from build123d import *

# Parameters (mm, degrees)
EXTRU_MINCE1_DEPTH      = 38
BOSS_EXTRU_1_DEPTH      = 1.2
CONG_1_R                = 1
BOSS_EXTRU_2_DEPTH      = 12
ESQUISSE4_R             = 1.5
ENL_V_MAT_EXTRU_1_DEPTH = 68.523625665
ESQUISSE5_W             = 8.01820663
ESQUISSE5_H             = 8
ENL_V_MAT_EXTRU_2_DEPTH = 10
CONG_2_R                = 3


with BuildPart() as part:
    # Esquisse1 → Extru.-Mince1 (new body)
    with BuildSketch(Plane(origin=(0, 0, 0), x_dir=(1, 0, 0), z_dir=(0, 1, 0))):
        with BuildLine():
            ThreePointArc((19.5687881, -17.869318182), (0, 26.5), (-19.5687881, -17.869318182))
            ThreePointArc((-19.5687881, -17.869318182), (0, -2), (19.5687881, -17.869318182))
        make_face()
        with BuildLine():
            ThreePointArc((20.124375889, -15.332954545), (0, 25.3), (-20.124375889, -15.332954545))
            ThreePointArc((-20.124375889, -15.332954545), (0, -0.8), (20.124375889, -15.332954545))
        make_face(mode=Mode.SUBTRACT)
    extrude(amount=EXTRU_MINCE1_DEPTH)

    # Esquisse2 → Boss.-Extru.1 (add)
    with BuildSketch(Plane(origin=(0, 0, 0), x_dir=(1, 0, 0), z_dir=(0, 1, 0))):
        with BuildLine():
            Line((-19.5687881, -17.869318182), (-24.368679521, -22.252358491))
            ThreePointArc((-24.368679521, -22.252358491), (0, 33), (24.368679521, -22.252358491))
            Line((24.368679521, -22.252358491), (19.5687881, -17.869318182))
            ThreePointArc((19.5687881, -17.869318182), (0, 26.5), (-19.5687881, -17.869318182))
        make_face()
    extrude(amount=BOSS_EXTRU_1_DEPTH)

    # Congé1
    cong_1_edges = [part.edges().sort_by_distance(p)[0] for p in [
        (-19.5687881, 19.6, 17.869318182),
        (19.5687881, 19.6, 17.869318182),
        (-20.124375889, 19, 15.332954545),
        (20.124375889, 19, 15.332954545),
    ]]
    fillet(cong_1_edges, radius=CONG_1_R)

    # Esquisse3 → Boss.-Extru.2 (add)
    with BuildSketch(Plane(origin=(0, 38, 0), x_dir=(1, 0, 0), z_dir=(0, 1, 0))):
        with BuildLine():
            ThreePointArc((20.241103191, -15.696212121), (19.846650871, -16.447482623), (19.095380369, -16.053030303))
            ThreePointArc((19.095380369, -16.053030303), (0, -2), (-19.095380369, -16.053030303))
            ThreePointArc((-19.095380369, -16.053030303), (-19.846650871, -16.447482623), (-20.241103191, -15.696212121))
            ThreePointArc((-20.241103191, -15.696212121), (0, -0.8), (20.241103191, -15.696212121))
        make_face()
    extrude(amount=BOSS_EXTRU_2_DEPTH)

    # Esquisse4 → Enlèv. mat.-Extru.1 (cut, through all)
    with BuildSketch(Plane(origin=(0, 1.2, 0), x_dir=(1, 0, 0), z_dir=(0, 1, 0))):
        with Locations(Location((-25.980762114, -15, 0), (0, 0, 270))):
            Circle(ESQUISSE4_R)
        with Locations(Location((0, 30, 0), (0, 0, 270))):
            Circle(ESQUISSE4_R)
        with Locations(Location((25.980762114, -15, 0), (0, 0, 270))):
            Circle(ESQUISSE4_R)
    extrude(amount=-ENL_V_MAT_EXTRU_1_DEPTH, mode=Mode.SUBTRACT)

    # Esquisse5 → Enlèv. mat.-Extru.2 (cut)
    with BuildSketch(Plane.XZ):
        with Locations((28.990896685, 0)):
            Rectangle(ESQUISSE5_W, ESQUISSE5_H)
    extrude(amount=-ENL_V_MAT_EXTRU_2_DEPTH, mode=Mode.SUBTRACT)

    # Congé2
    cong_2_edges = [part.edges().sort_by_distance(p)[0] for p in [
        (25.589083583, 10, 4),
        (32.756678708, 0.6, 4),
        (25.589083583, 10, -4),
        (32.756678708, 0.6, -4),
        (-19.5687881, 0.6, 17.869318182),
        (19.5687881, 0.6, 17.869318182),
        (24.368679521, 0.6, 22.252358491),
        (-24.368679521, 0.6, 22.252358491),
    ]]
    fillet(cong_2_edges, radius=CONG_2_R)


solid = part.part
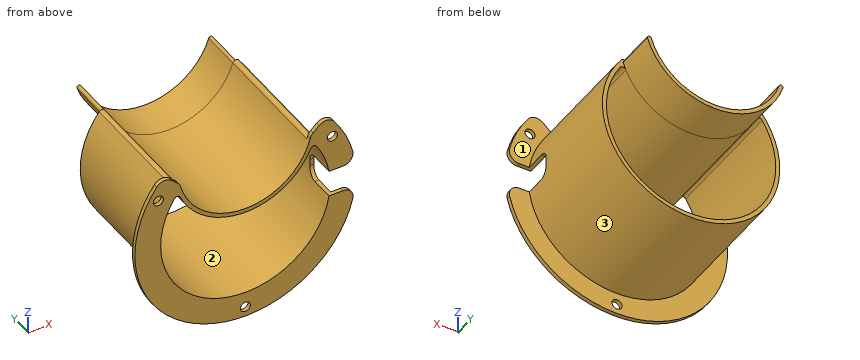
CAD build for the part. Positions are in the model's coordinates, mm. Face numbers are marked on the shaded views. Round coordinates to 2 decimals unless told otherwise and drop trailing zeros. Loops run counter-clockwise (first coordinate to the right, second up) from the corner with the lowest first, then second, coordinate; pieces in that order, holes last. Notation, with made-up numbers: (19.5, 34.25) - (65.5, 34.25) arc R15 ccw to (65.5, 55.25) - close; hole circle Ø7 at (20.25, -23.75). An arc over 180 degrees is marked (long way). Put each result on its own line as item: value.
1. Slice it at C-C on z = 8.5. List the corners of the cut face in (x, y).
Geometry check:
outline: (-31.89, 0) - (-23.83, 0) - (-23.83, 38) - (-25.1, 38) - (-25.1, 1.2) - (-31.89, 1.2) - close; (-16.35, 0) - (-14.76, 0) - (-14.76, 50) - (-16.35, 50) - close; (14.76, 0) - (16.35, 0) - (16.35, 50) - (14.76, 50) - close; (23.83, 0) - (31.89, 0) - (31.89, 1.2) - (25.1, 1.2) - (25.1, 38) - (23.83, 38) - close
2. Two-plate mould, pull along Z, no slides. Class the marked faces 1, 2 and 3: released by +Z, released by -Z, zero draft, split by the parting line, or undercut.
Geometry check:
face 1: zero draft
face 2: undercut
face 3: split by the parting line
3. Slice it at B-B on x = 0. List the corners of the cut face in (y, z).
Geometry check:
outline: (0, -33) - (1.2, -33) - (1.2, -31.5) - (0, -31.5) - close; (0, -28.5) - (1.2, -28.5) - (1.2, -26.5) - (38, -26.5) - (38, -25.3) - (0, -25.3) - close; (0, 0.8) - (50, 0.8) - (50, 2) - (0, 2) - close
4. Slice it at A-A on z = 0. List the corners of the cut face in (x, y), and give its area (3 significant figures).
Geometry check:
outline: (-33, 0) - (-25.3, 0) - (-25.3, 38) - (-26.5, 38) - (-26.5, 1.2) - (-33, 1.2) - close; (25.3, 10) - (26.5, 10) - (26.5, 38) - (25.3, 38) - close
area: 87.0 mm²
5. Wall check: line 1 (X direction, y = 0.75, z = 15) (3 decimals); line 2 (X direction, y = 22, z = 0); line 3 (X direction, y = 21.5, z = 9). Give the ranges that are in metal, low to high.
Geometry check:
line 1: -29.394 to -27.481, -24.481 to -18.735, 18.735 to 24.481, 27.481 to 29.394
line 2: -26.5 to -25.3, 25.3 to 26.5
line 3: -24.92 to -23.65, -16.75 to -15.2, 15.2 to 16.75, 23.65 to 24.92
6. Slice it at D-D on x = -16.5. List the corners of the cut face in (y, z).
Geometry check:
outline: (0, -28.58) - (1.2, -28.58) - (1.2, -20.74) - (38, -20.74) - (38, -19.18) - (0, -19.18) - close; (0, 8.69) - (50, 8.69) - (50, 10.7) - (0, 10.7) - close
7. Pin check, flat tips, straight feed: P1, Ø4, axis at x = -24, y = 30.5, coming from the +Z side; P2, Ø4, axis at x = 25.98, z = 15, coming from the +Y side; P3, Ø4, axis at x = 23.5, z = 10.5, coming from the +Y side; P4, Ø3.5, axis at x = 0, z = -30, coming from the -Y side. Stop position of each tip, or through.
Geometry check:
P1: z = 14.77
P2: y = 1.2
P3: y = 38
P4: y = 0
